```python
from build123d import *

# Parameters (mm, degrees)
SKETCH_1_R          = 1
SKETCH_1_R_2        = 1.65
SKETCH_1_R_3        = 10
EXTRUDE_2_DEPTH     = 5
CUT_EXTRUDE_1_DEPTH = 5
SKETCH_4_R          = 1.65
CUT_EXTRUDE_3_DEPTH = 5
SKETCH_5_R          = 1.65
CUT_EXTRUDE_4_DEPTH = 5


with BuildPart() as part:
    # 草图1 → 凸台-拉伸2 (new body)
    with BuildSketch(Plane(origin=(0, 0, 0), x_dir=(1, 0, 0), z_dir=(0, 1, 0))):
        with BuildLine():
            Line((-43.8590831, 198.080740626), (-16.3590831, 198.080740626))
            Line((-16.3590831, 198.080740626), (-16.3590831, 138.080740626))
            ThreePointArc((-16.3590831, 138.080740626), (-13.430150911, 131.009672814), (-6.3590831, 128.080740626))
            Line((-6.3590831, 128.080740626), (48.6409169, 128.080740626))
            ThreePointArc((48.6409169, 128.080740626), (55.711984712, 131.009672814), (58.6409169, 138.080740626))
            Line((58.6409169, 138.080740626), (58.6409169, 198.080740626))
            Line((58.6409169, 198.080740626), (86.1409169, 198.080740626))
            ThreePointArc((86.1409169, 198.080740626), (93.211984712, 195.151808438), (96.1409169, 188.080740626))
            Line((96.1409169, 188.080740626), (96.1409169, 133.080740626))
            Line((96.1409169, 133.080740626), (86.1409169, 133.080740626))
            Line((86.1409169, 133.080740626), (86.1409169, 73.080740626))
            Line((86.1409169, 73.080740626), (108.1409169, 73.080740626))
            Line((108.1409169, 73.080740626), (108.1409169, -1.919259374))
            Line((108.1409169, -1.919259374), (86.1409169, -1.919259374))
            Line((86.1409169, -1.919259374), (86.1409169, -61.919259374))
            Line((86.1409169, -61.919259374), (95.08518881, -61.919259374))
            ThreePointArc((95.08518881, -61.919259374), (95.830544803, -62.252592707), (96.0789968, -63.030370485))
            ThreePointArc((96.0789968, -63.030370485), (92.807583567, -69.372819299), (86.1409169, -71.919259374))
            Line((86.1409169, -71.919259374), (38.4459169, -71.919259374))
            Line((38.4459169, -71.919259374), (38.4459169, -59.419259374))
            Line((38.4459169, -59.419259374), (15.4159169, -59.419259374))
            Line((15.4159169, -59.419259374), (15.4159169, -71.919259374))
            Line((15.4159169, -71.919259374), (-43.8590831, -71.919259374))
            ThreePointArc((-43.8590831, -71.919259374), (-50.525749766, -69.372819299), (-53.797163, -63.030370485))
            ThreePointArc((-53.797163, -63.030370485), (-53.548711002, -62.252592707), (-52.80335501, -61.919259374))
            Line((-52.80335501, -61.919259374), (-43.8590831, -61.919259374))
            Line((-43.8590831, -61.919259374), (-43.8590831, -1.919259374))
            Line((-43.8590831, -1.919259374), (-65.8590831, -1.919259374))
            Line((-65.8590831, -1.919259374), (-65.8590831, 73.080740626))
            Line((-65.8590831, 73.080740626), (-43.8590831, 73.080740626))
            Line((-43.8590831, 73.080740626), (-43.8590831, 133.080740626))
            Line((-43.8590831, 133.080740626), (-53.8590831, 133.080740626))
            Line((-53.8590831, 133.080740626), (-53.8590831, 188.080740626))
            ThreePointArc((-53.8590831, 188.080740626), (-50.930150911, 195.151808438), (-43.8590831, 198.080740626))
        make_face()
        with Locations(Location((13.0959169, -65.669259374, 0), (0, 0, 270))):
            Circle(SKETCH_1_R, mode=Mode.SUBTRACT)
        with Locations(Location((40.7659169, -65.669259374, 0), (0, 0, 270))):
            Circle(SKETCH_1_R, mode=Mode.SUBTRACT)
        with Locations(Location((66.1409169, 17.080740626, 0), (0, 0, 90))):
            Circle(SKETCH_1_R_2, mode=Mode.SUBTRACT)
        with Locations(Location((-60.8590831, 54.080740626, 0), (0, 0, 270))):
            Circle(SKETCH_1_R_2, mode=Mode.SUBTRACT)
        with Locations(Location((-23.8590831, 54.080740626, 0), (0, 0, 270))):
            Circle(SKETCH_1_R_2, mode=Mode.SUBTRACT)
        with Locations(Location((-23.8590831, 17.080740626, 0), (0, 0, 270))):
            Circle(SKETCH_1_R_2, mode=Mode.SUBTRACT)
        with Locations(Location((-60.8590831, 17.080740626, 0), (0, 0, 270))):
            Circle(SKETCH_1_R_2, mode=Mode.SUBTRACT)
        with Locations(Location((103.1409169, 17.080740626, 0), (0, 0, 90))):
            Circle(SKETCH_1_R_2, mode=Mode.SUBTRACT)
        with Locations(Location((103.1409169, 54.080740626, 0), (0, 0, 90))):
            Circle(SKETCH_1_R_2, mode=Mode.SUBTRACT)
        with Locations(Location((66.1409169, 54.080740626, 0), (0, 0, 90))):
            Circle(SKETCH_1_R_2, mode=Mode.SUBTRACT)
        with Locations(Location((-38.8590831, 111.080740626, 0), (0, 0, 270))):
            Circle(SKETCH_1_R_2, mode=Mode.SUBTRACT)
        with Locations(Location((-24.8590831, 111.080740626, 0), (0, 0, 270))):
            Circle(SKETCH_1_R_2, mode=Mode.SUBTRACT)
        with Locations(Location((-24.8590831, 95.080740626, 0), (0, 0, 270))):
            Circle(SKETCH_1_R_2, mode=Mode.SUBTRACT)
        with Locations(Location((-38.8590831, 95.080740626, 0), (0, 0, 270))):
            Circle(SKETCH_1_R_2, mode=Mode.SUBTRACT)
        with Locations(Location((-38.8590831, -23.919259374, 0), (0, 0, 270))):
            Circle(SKETCH_1_R_2, mode=Mode.SUBTRACT)
        with Locations(Location((-24.8590831, -23.919259374, 0), (0, 0, 270))):
            Circle(SKETCH_1_R_2, mode=Mode.SUBTRACT)
        with Locations(Location((-38.8590831, -39.919259374, 0), (0, 0, 270))):
            Circle(SKETCH_1_R_2, mode=Mode.SUBTRACT)
        with Locations(Location((-24.8590831, -39.919259374, 0), (0, 0, 270))):
            Circle(SKETCH_1_R_2, mode=Mode.SUBTRACT)
        with Locations(Location((-29.0090831, 184.430740626, 0), (0, 0, 270))):
            Circle(SKETCH_1_R_2, mode=Mode.SUBTRACT)
        with Locations(Location((-42.7090831, 184.430740626, 0), (0, 0, 270))):
            Circle(SKETCH_1_R_2, mode=Mode.SUBTRACT)
        with Locations(Location((-42.7090831, 146.730740626, 0), (0, 0, 270))):
            Circle(SKETCH_1_R_2, mode=Mode.SUBTRACT)
        with Locations(Location((-29.0090831, 146.730740626, 0), (0, 0, 270))):
            Circle(SKETCH_1_R_2, mode=Mode.SUBTRACT)
        with Locations(Location((-24.8590831, 128.080740626, 0), (0, 0, 270))):
            Circle(SKETCH_1_R_2, mode=Mode.SUBTRACT)
        with Locations(Location((-9.8590831, -51.919259374, 0), (0, 0, 270))):
            Circle(SKETCH_1_R_2, mode=Mode.SUBTRACT)
        with Locations(Location((52.1409169, -51.919259374, 0), (0, 0, 90))):
            Circle(SKETCH_1_R_2, mode=Mode.SUBTRACT)
        with Locations(Location((67.1409169, -39.919259374, 0), (0, 0, 90))):
            Circle(SKETCH_1_R_2, mode=Mode.SUBTRACT)
        with Locations(Location((81.1409169, -39.919259374, 0), (0, 0, 90))):
            Circle(SKETCH_1_R_2, mode=Mode.SUBTRACT)
        with Locations(Location((67.1409169, -23.919259374, 0), (0, 0, 90))):
            Circle(SKETCH_1_R_2, mode=Mode.SUBTRACT)
        with Locations(Location((81.1409169, -23.919259374, 0), (0, 0, 90))):
            Circle(SKETCH_1_R_2, mode=Mode.SUBTRACT)
        with Locations(Location((81.1409169, 95.080740626, 0), (0, 0, 90))):
            Circle(SKETCH_1_R_2, mode=Mode.SUBTRACT)
        with Locations(Location((67.1409169, 95.080740626, 0), (0, 0, 90))):
            Circle(SKETCH_1_R_2, mode=Mode.SUBTRACT)
        with Locations(Location((67.1409169, 111.080740626, 0), (0, 0, 90))):
            Circle(SKETCH_1_R_2, mode=Mode.SUBTRACT)
        with Locations(Location((81.1409169, 111.080740626, 0), (0, 0, 90))):
            Circle(SKETCH_1_R_2, mode=Mode.SUBTRACT)
        with Locations(Location((67.1409169, 128.080740626, 0), (0, 0, 90))):
            Circle(SKETCH_1_R_2, mode=Mode.SUBTRACT)
        with Locations(Location((71.2909169, 146.730740626, 0), (0, 0, 90))):
            Circle(SKETCH_1_R_2, mode=Mode.SUBTRACT)
        with Locations(Location((84.9909169, 146.730740626, 0), (0, 0, 90))):
            Circle(SKETCH_1_R_2, mode=Mode.SUBTRACT)
        with Locations(Location((84.9909169, 184.430740626, 0), (0, 0, 90))):
            Circle(SKETCH_1_R_2, mode=Mode.SUBTRACT)
        with Locations(Location((71.2909169, 184.430740626, 0), (0, 0, 90))):
            Circle(SKETCH_1_R_2, mode=Mode.SUBTRACT)
        with Locations(Location((21.1409169, 64.080740626, 0), (0, 0, 270))):
            Circle(SKETCH_1_R_3, mode=Mode.SUBTRACT)
    extrude(amount=EXTRUDE_2_DEPTH)

    # 草图2 → 切除-拉伸1 (cut)
    with BuildSketch(Plane(origin=(0, 5, 0), x_dir=(1, 0, 0), z_dir=(0, 1, 0))):
        with BuildLine():
            Line((52.7909169, 118.080740626), (52.7909169, 103.080740626))
            ThreePointArc((52.7909169, 103.080740626), (51.1409169, 101.430740626), (49.4909169, 103.080740626))
            Line((49.4909169, 103.080740626), (49.4909169, 118.080740626))
            ThreePointArc((49.4909169, 118.080740626), (51.1409169, 119.730740626), (52.7909169, 118.080740626))
        make_face()
        with BuildLine():
            Line((-7.2090831, 118.080740626), (-7.2090831, 103.080740626))
            ThreePointArc((-7.2090831, 103.080740626), (-8.8590831, 101.430740626), (-10.5090831, 103.080740626))
            Line((-10.5090831, 103.080740626), (-10.5090831, 118.080740626))
            ThreePointArc((-10.5090831, 118.080740626), (-8.8590831, 119.730740626), (-7.2090831, 118.080740626))
        make_face()
    extrude(amount=-CUT_EXTRUDE_1_DEPTH, mode=Mode.SUBTRACT)

    # 草图4 → 切除-拉伸3 (cut)
    with BuildSketch(Plane.XZ):
        with Locations(Location((-31.8590831, 31.919259374, 0), (0, 0, 270))):
            Circle(SKETCH_4_R)
        with Locations(Location((-31.8590831, 54.919259374, 0), (0, 0, 270))):
            Circle(SKETCH_4_R)
        with Locations(Location((74.1409169, 31.919259374, 0), (0, 0, 270))):
            Circle(SKETCH_4_R)
        with Locations(Location((74.1409169, 54.919259374, 0), (0, 0, 270))):
            Circle(SKETCH_4_R)
    extrude(amount=-CUT_EXTRUDE_3_DEPTH, mode=Mode.SUBTRACT)

    # 草图5 → 切除-拉伸4 (cut)
    with BuildSketch(Plane.XZ):
        with Locations(Location((93.1409169, -65.580740626, 0), (0, 0, 270))):
            Circle(SKETCH_5_R)
        with Locations(Location((93.1409169, -5.580740626, 0), (0, 0, 270))):
            Circle(SKETCH_5_R)
        with Locations(Location((-50.8590831, -5.580740626, 0), (0, 0, 90))):
            Circle(SKETCH_5_R)
        with Locations(Location((-50.8590831, -65.580740626, 0), (0, 0, 90))):
            Circle(SKETCH_5_R)
    extrude(amount=-CUT_EXTRUDE_4_DEPTH, mode=Mode.SUBTRACT)


solid = part.part
```
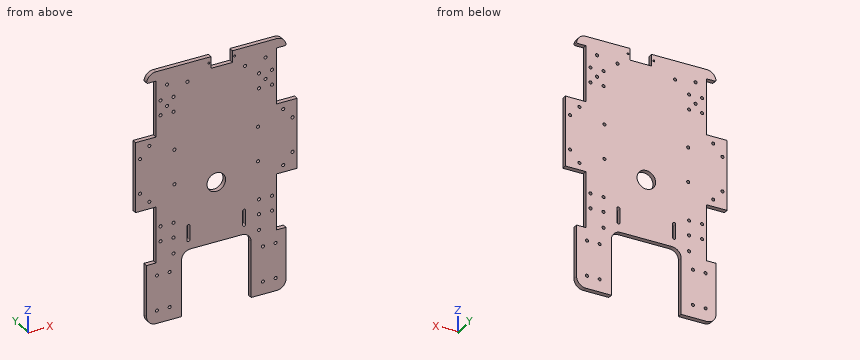
Geometry: final body of the model. Coordinates: model frame, mm. Coordinates: 2 decimals unless noted, no trailing zeros. Order: outer loops, then holes, each group sorted by start corner. A loop starts at its lowest first (then second) coordinate and runs counter-clockwise, first axis right, second up. Notation, with made-up numbers: (2.5, 31.5) - (26.5, 31.5) arc R20 ccw to (26.5, 60.5) - close; hole circle Ø1 at (29.25, 0). An arc over 180 degrees is marked (long way). Return JSON: item names as keys, results as strings. Group by question number.
1. Pin query (flat end, axial travel): pin 1 (3 mm diameter, centred on x = 93.14, z = -65.58, fed in from +Y) (3 decimals); pin 2 (3 mm diameter, centred on y = 3.5, z = -150, fed in from +X); pin 3 (2.5 mm diameter, centred on y = 1.5, z = -156.5, fed in from -X); pin 4 (2.5 mm diameter, centred on x = 23, y = 3.5, fed in from +Z). Return the tip coordinate at first contact, or that it passes through.
2. Cut plane A-A (z = -172.5). Output: boundary loops of the cut face in (x, y).
3. Cut plane B-B (y = 2.55). Count the separate pieces of the cut face and the enclosed holes in it, plus the area to 3 significant figures.
4. Material intervals for line 1 along X through (y, z) = (2, -115.5); line 2 along X through (y, z) = (2.6, -182.5); line 3 along Z through (x, y) = (-26, 3.85), sorted ascending. Write a range as [from, to].
Resolved:
{
 "1": {"pin 1": "passes through", "pin 2": "stops at x = 96.14", "pin 3": "stops at x = -53.86", "pin 4": "stops at z = 59.42"},
 "2": {"outline": "(-53.86, 0) - (-16.36, 0) - (-16.36, 5) - (-53.86, 5) - close; (58.64, 0) - (96.14, 0) - (96.14, 5) - (58.64, 5) - close"},
 "3": {"separate pieces": "1", "enclosed holes": "49", "area": "33,500 mm²"},
 "4": {"line 1": "x = [-43.86, -10.51], [-7.21, 49.49], [52.79, 86.14]", "line 2": "x = [-53.86, -16.36], [58.64, 96.14]", "line 3": "z = [-198.08, -129.27], [-126.89, -112.27], [-109.89, -96.27], [-93.89, 22.73], [25.11, 38.73], [41.11, 71.92]"}
}
